Model file for the job. Use its own axes, mm. A direction names the side the tool comes from. Coordinates: 2 decimals unless noted, no trailing zeros. Order: outer loops, then holes, each group sorted by start corner. A loop starts at its lowest first (then second) coordinate and runs counter-clockwise, first axis right, second up. Notation, with made-up numbers: (44, -1) -> (98, -1) arc R27 cw to (98, 27) -> close; hole circle Ø4 at (-22.75, 38). An arc over 180 degrees is marked (long way). Use CSV: the item, a comma, the result in double quotes. Start each with the question number.
(1) Pull direction Y, two halves, no side cores. Call faces 6 (the conical face through (-96.74, 96.89, 3.86)), 7 (the cylindrical face through (-97.15, -96.99, 1.98)), 8 (the cylindrical face through (-98.63, 10.64, 1.98)): pulls with the +Y half, pulls with the -Y half, needs draft (parallel to the pull), parting line crosses it, or undercut.
(2) Cut at A-A on y = 5.5. Write the cut outline in (x, z), plus the area to 4 significant figures.
(3) Probe L1, parallel to Y at x = -81.5, z = 3.1; L2, parallel to Y at x = -20, z = 0.4; L3, parallel to Y at x = 90.5, z = 2.9. List the from-to ranges inside material, lowest first.
(4) Tool access for faces 1 (the conical face through (-98.302, -10.829, 3.865)), 2 (the cylindrical face through (-98.56, -10.57, 1.98)), 3 (the conical face through (-96.74, 96.89, 0.14)), 4 (the cylindrical face through (-96.99, 97.15, 1.98)), 5 (the conical face through (-98.371, 10.898, 0.135)): list every direction of +Z, -Z, +X, -X, +Y, -Y with a clear straight run to the whole face (end or side of a thin tool).
```python
from build123d import *

# Parameters (mm, degrees)
F1_DEPTH = 4
F2_SIZE  = 0.5


with BuildPart() as f1:
    # F0 (on Top) → F1 (new body)
    with BuildSketch(Plane.XY):
        with BuildLine():
            Line((-90, -100), (90, -100))
            ThreePointArc((90, -100), (97.071068, -97.071068), (100, -90))
            Line((100, -90), (100, 90))
            ThreePointArc((100, 90), (97.071068, 97.071068), (90, 100))
            Line((90, 100), (-90, 100))
            ThreePointArc((-90, 100), (-97.071068, 97.071068), (-100, 90))
            Line((-100, 90), (-100, 14))
            ThreePointArc((-100, 14), (-98.594113, 10.605887), (-95.2, 9.2))
            Line((-95.2, 9.2), (-80, 9.2))
            Line((-80, 9.2), (-80, -9.2))
            Line((-80, -9.2), (-95.2, -9.2))
            ThreePointArc((-95.2, -9.2), (-98.594113, -10.605887), (-100, -14))
            Line((-100, -14), (-100, -90))
            ThreePointArc((-100, -90), (-97.071068, -97.071068), (-90, -100))
        make_face()
    extrude(amount=F1_DEPTH)

    # F2
    f2_edges = [f1.edges().sort_by_distance(p)[0] for p in [
        (0, -100, 4),
        (97.071068, -97.071068, 4),
        (100, 0, 4),
        (97.071068, 97.071068, 4),
        (0, 100, 4),
        (-97.071068, 97.071068, 4),
        (-100, 52, 4),
        (-98.594113, 10.605887, 4),
        (-87.6, 9.2, 4),
        (-80, 0, 4),
        (-87.6, -9.2, 4),
        (-98.594113, -10.605887, 4),
        (-100, -52, 4),
        (-97.071068, -97.071068, 4),
        (0, -100, 0),
        (97.071068, -97.071068, 0),
        (100, 0, 0),
        (97.071068, 97.071068, 0),
        (0, 100, 0),
        (-97.071068, 97.071068, 0),
        (-100, 52, 0),
        (-98.594113, 10.605887, 0),
        (-87.6, 9.2, 0),
        (-80, 0, 0),
        (-87.6, -9.2, 0),
        (-98.594113, -10.605887, 0),
        (-100, -52, 0),
        (-97.071068, -97.071068, 0),
    ]]
    chamfer(f2_edges, length=F2_SIZE)


solid = f1.part
```
Outcome:
1,face 6,"pulls with the +Y half"
1,face 7,"pulls with the -Y half"
1,face 8,"undercut"
2,outline,"(-80, 0.5) -> (-79.5, 0) -> (99.5, 0) -> (100, 0.5) -> (100, 3.5) -> (99.5, 4) -> (-79.5, 4) -> (-80, 3.5) -> close"
2,area,"719.5 mm2"
3,L1,"-100 to -9.2, 9.2 to 100"
3,L2,"-99.9 to 99.9"
3,L3,"-99.99 to 99.99"
4,face 1,"+Z, -X"
4,face 2,"+Z, -Z, -X"
4,face 3,"-Z, -X, +Y"
4,face 4,"+Z, -Z, -X, +Y"
4,face 5,"-Z, -X"
